Autodesk Inventor part; units mm, degrees
ref_plane "YZ Plane" through (0, 0, 0) normal (1, 0, 0) x (0, 1, 0)
ref_plane "XZ Plane" through (0, 0, 0) normal (0, 1, 0) x (-1, 0, 0)
ref_plane "XY Plane" through (0, 0, 0) normal (0, 0, 1) x (1, 0, 0)
sketch "Sketch1" plane through (0, 0, 0) normal (0, 1, 0) x (-1, 0, 0)
  circle A0 centre (0, 0) radius 20.5
  circle A1 centre (0, 0) radius 23
  dimension "d2" = 41
  dimension "d3" = 46
extrude "Extrusion1" add sketch "Sketch1" along normal mid plane 10
sketch "Sketch2" plane through (0, 0, 0) normal (1, 0, 0) x (0, 1, 0)
  circle A0 centre (0, 0) radius 2
  dimension "d6" = 4
extrude "Extrusion2" cut sketch "Sketch2" along normal through all both and the other way through all
sketch "Sketch3" plane through (0, 0, 0) normal (0, 0, 1) x (1, 0, 0)
  circle A0 centre (0, 0) radius 2
  dimension "d9" = 4
extrude "Extrusion3" cut sketch "Sketch3" along normal through all both and the other way through all
Can you work these out from the model? Positions are in its coordinate system, mm. Give positions to 0.01 mm unless a question says otherwise; leave off trailing zeros. Order: outer loops, then holes, each group sorted by start corner. A loop starts at its lowest first (then second) coordinate and runs counter-clockwise, first axis right, second up. Notation, with made-up numbers: M 27,24.5 L 47,24.5 A12 cw 47,47.5 Z; hole C -8.75,55 d11. An arc over 180 degrees is marked long. One line per question, with ' | ' between items.
Item 1: Suppose I cut it at A-A, the plane z = 0. Write out the boundary of the cut face in (x, y), then the cut area to 3 significant figures.
Answer block:
outline: M -23,-5 L -20.5,-5 L -20.5,-2 L -23,-2 Z; M -23,2 L -20.5,2 L -20.5,5 L -23,5 Z; M 20.5,-5 L 23,-5 L 23,-2 L 20.5,-2 Z; M 20.5,2 L 23,2 L 23,5 L 20.5,5 Z | area: 30.0 mm2
Item 2: I'm going to push flat-ended pins straight in: pin 1 Ø6 at (x, y) = (14.5, -3.5) entering from +Z; pin 2 Ø6 at (y, z) = (0, 8) entering from +X; pin 3 Ø3 at (y, z) = (1.5, -13.5) entering from -X; pin 4 Ø2.5 at (x, y) = (0, 0) entering from -Z. Where does each tip first touch, or does it pass through?
Answer block:
pin 1: stops at z = 19.92 | pin 2: stops at x = 22.45 | pin 3: stops at x = -19.62 | pin 4: passes through
Item 3: Please list where these lines run through material, in increasing order: L1, parallel to Y at x = 0, z = -21.1; L2, parallel to Z at x = -1, y = 2.25; L3, parallel to Z at x = -11.5, y = 2.
Answer block:
L1: y = -5 to -2, 2 to 5 | L2: z = -22.98 to -20.48, 20.48 to 22.98 | L3: z = -19.92 to -16.97, 16.97 to 19.92
Item 4: Suppose I cut it at C-C, the plane x = 13.5. Write out the boundary of the cut face in (y, z), then the cut area to 3 significant figures.
Answer block:
outline: M -5,-18.62 L 5,-18.62 L 5,-15.43 L -5,-15.43 Z; M -5,15.43 L 5,15.43 L 5,18.62 L -5,18.62 Z | area: 63.9 mm2
Item 5: Suppose I cut it at D-D, the plane y = 3.25. Write out the boundary of the cut face in (x, z).
Answer block:
outline: C 0,0 d46; hole C 0,0 d41
Item 6: Suppose I cut it at B-B, the plane x = 0. Write out the boundary of the cut face in (y, z).
Answer block:
outline: M -5,-23 L -2,-23 L -2,-20.5 L -5,-20.5 Z; M -5,20.5 L -2,20.5 L -2,23 L -5,23 Z; M 2,-23 L 5,-23 L 5,-20.5 L 2,-20.5 Z; M 2,20.5 L 5,20.5 L 5,23 L 2,23 Z
Item 7: We'd pull the mould along Z, two halves only. Please class faces 1 (the face through (22, 0, 2)), 2 (the face through (-21.938, -0.07, -6.909)), 3 (the face through (0, -2, -22)): released by +Z, released by -Z, zero draft, split by the parting line, or undercut.
Answer block:
face 1: undercut | face 2: split by the parting line | face 3: zero draft
